from build123d import *

# Parameters (mm, degrees)
SKETCH1_W            = 75
SKETCH1_H            = 40
BOSS_EXTRUDE1_DEPTH  = 2
SKETCH2_W            = 75
SKETCH2_H            = 40
SKETCH2_W_2          = 71
SKETCH2_H_2          = 17
BOSS_EXTRUDE2_DEPTH  = 17
CUT_EXTRUDE2_DEPTH   = 17
CUT_EXTRUDE3_REACH   = 82.169
CUT_EXTRUDE4_REACH   = 88.683
SKETCH5_R            = 1.6
MIRROR2_COPY_1_DEPTH = 17
SKETCH7_W            = 80.259890461
SKETCH7_H            = 23.370696072
CUT_EXTRUDE5_DEPTH   = 19


with BuildPart() as part:
    # Sketch1 → Boss-Extrude1 (new body)
    with BuildSketch(Plane(origin=(0, 0, 0), x_dir=(1, 0, 0), z_dir=(0, 1, 0))):
        with Locations((37.5, 20)):
            Rectangle(SKETCH1_W, SKETCH1_H)
    boss_extrude1 = extrude(amount=BOSS_EXTRUDE1_DEPTH)

    # Sketch2 → Boss-Extrude2 (add)
    with BuildSketch(Plane(origin=(0, 2, 0), x_dir=(1, 0, 0), z_dir=(0, 1, 0))):
        with Locations((37.5, 20)):
            Rectangle(SKETCH2_W, SKETCH2_H)
        with Locations((37.5, 29.5)):
            Rectangle(SKETCH2_W_2, SKETCH2_H_2, mode=Mode.SUBTRACT)
        with Locations((37.5, 10.5)):
            Rectangle(SKETCH2_W_2, SKETCH2_H_2, mode=Mode.SUBTRACT)
    boss_extrude2 = extrude(amount=BOSS_EXTRUDE2_DEPTH)

    # Sketch3 → Cut-Extrude2 (cut)
    with BuildSketch(Plane.XY):
        with BuildLine():
            Line((2, 17.5), (2, 19))
            Line((2, 19), (73, 19))
            Line((73, 19), (73, 17.5))
            ThreePointArc((73, 17.5), (70.5, 15), (68, 17.5))
            Line((68, 17.5), (49, 17.5))
            Line((49, 17.5), (46, 15))
            Line((46, 15), (29, 15))
            Line((29, 15), (26, 17.5))
            Line((26, 17.5), (7, 17.5))
            ThreePointArc((7, 17.5), (4.5, 15), (2, 17.5))
        make_face()
    cut_extrude2 = extrude(amount=-CUT_EXTRUDE2_DEPTH, mode=Mode.SUBTRACT)

    # Mirror1: Cut-Extrude2 across plane
    add(cut_extrude2.mirror(Plane.XY.offset(-20)), mode=Mode.SUBTRACT)

    # Sketch4 → Cut-Extrude3 (cut, up to next)
    with BuildSketch(Plane.XY.offset(-19), mode=Mode.PRIVATE) as cut_extrude3_sk1:
        Polygon((2, 18), (7.035918341, 18), (10.035918341, 15), (64.964081659, 15), (67.964081659, 18), (73, 18), (73, 19), (2, 19), align=None)
    cut_extrude3_tool1 = extrude(cut_extrude3_sk1.sketch, amount=-CUT_EXTRUDE3_REACH, mode=Mode.PRIVATE) & part.part
    cut_extrude3 = cut_extrude3_tool1.solids().sort_by_distance((37.5, 17.098486, -19))[0]
    add(cut_extrude3, mode=Mode.SUBTRACT)

    # Sketch5 → Cut-Extrude4 (cut, up to next)
    with BuildSketch(Plane(origin=(0, 2, 0), x_dir=(1, 0, 0), z_dir=(0, 1, 0)), mode=Mode.PRIVATE) as cut_extrude4_sk1:
        with Locations(Location((37.5, 29.5, 0), (0, 0, 270))):
            Circle(SKETCH5_R)
    cut_extrude4_tool1 = extrude(cut_extrude4_sk1.sketch, amount=-CUT_EXTRUDE4_REACH, mode=Mode.PRIVATE) & part.part
    # Sketch5 → Cut-Extrude4 (cut, up to next)
    with BuildSketch(Plane(origin=(0, 2, 0), x_dir=(1, 0, 0), z_dir=(0, 1, 0)), mode=Mode.PRIVATE) as cut_extrude4_sk2:
        with Locations(Location((37.5, 10.5, 0), (0, 0, 270))):
            Circle(SKETCH5_R)
    cut_extrude4_tool2 = extrude(cut_extrude4_sk2.sketch, amount=-CUT_EXTRUDE4_REACH, mode=Mode.PRIVATE) & part.part
    cut_extrude4_1 = cut_extrude4_tool1.solids().sort_by_distance((37.5, 2, -29.5))[0]
    add(cut_extrude4_1, mode=Mode.SUBTRACT)
    cut_extrude4_2 = cut_extrude4_tool2.solids().sort_by_distance((37.5, 2, -10.5))[0]
    add(cut_extrude4_2, mode=Mode.SUBTRACT)
    cut_extrude4 = cut_extrude4_1 + cut_extrude4_2  # Cut-Extrude4 as one shape, for the pattern or mirror that repeats it

    # Mirror2: Boss-Extrude1, Boss-Extrude2, Cut-Extrude2, Cut-Extrude3, Cut-Extrude4 across plane
    add(boss_extrude1.mirror(Plane.XY.offset(-1)))
    add(boss_extrude2.mirror(Plane.XY.offset(-1)))
    add(cut_extrude2.mirror(Plane.XY.offset(-1)), mode=Mode.SUBTRACT)
    add(cut_extrude3.mirror(Plane.XY.offset(-1)), mode=Mode.SUBTRACT)
    add(cut_extrude4.mirror(Plane.XY.offset(-1)), mode=Mode.SUBTRACT)

    # Mirror2 copy 1 sketch → Mirror2 copy 1 (cut)
    with BuildSketch(Plane.XY.offset(38)):
        with BuildLine():
            Line((2, 17.5), (2, 19))
            Line((2, 19), (73, 19))
            Line((73, 19), (73, 17.5))
            ThreePointArc((73, 17.5), (70.5, 15), (68, 17.5))
            Line((68, 17.5), (49, 17.5))
            Line((49, 17.5), (46, 15))
            Line((46, 15), (29, 15))
            Line((29, 15), (26, 17.5))
            Line((26, 17.5), (7, 17.5))
            ThreePointArc((7, 17.5), (4.5, 15), (2, 17.5))
        make_face()
    extrude(amount=-MIRROR2_COPY_1_DEPTH, mode=Mode.SUBTRACT)

    # Sketch7 → Cut-Extrude5 (cut)
    with BuildSketch(Plane.XY.offset(38)):
        with Locations((37.807509159, 10.038141028)):
            Rectangle(SKETCH7_W, SKETCH7_H)
    extrude(amount=-CUT_EXTRUDE5_DEPTH, mode=Mode.SUBTRACT)


solid = part.part
For this review, take the finished solid that the model builds, in its own axes (mm). A direction names the side the tool comes from. Round coordinates to 2 decimals unless told otherwise and drop trailing zeros. Order: outer loops, then holes, each group sorted by start corner. A loop starts at its lowest first (then second) coordinate and runs counter-clockwise, first axis right, second up. Notation, with made-up numbers: M 65.5,51 L 81.5,51 A16 cw 81.5,80 Z; hole C -4.75,50 d4. An arc over 180 degrees is marked long. Use a Markdown table: item, result. Add a question column.
Item 1: Insertion check: pin 1 (0.6 mm diameter, centred on x = 62.5, z = -39, fed in from +Y); pin 2 (0.6 mm diameter, centred on x = 69.5, z = 18, fed in from +Y); pin 3 (8.5 mm diameter, centred on x = 51, z = -12.5, fed in from +Y). Each pin has a flat end and moves straight along its axis. Give the tip position at first contact, or say it passes through.
Item 2: Add section C-C, the plane z = -29.5. Give the boundary of the cut face in (x, y), then the cut area to 3 significant figures.
Item 3: Tool access review of faces 5 (the cylindrical face through (4.6, 15, -39)), 6 (the flat face through (66.443, 16.479, -19.986)), 7 (the cylindrical face through (35.94, 1.01, -29.85)), 8 (the flat face through (37, 7, -40)), 9 (the flat face through (70, 18, 18)): name each direction out of +Z, -Z, +X, -X, +Y, -Y from which nothing blocks a thin tool from reaching the whole face with its end or side.
Item 4: Add section D-D, the plane x = 4.5. Give the boundary of the cut face in (y, z).
Item 5: Add section B-B, the plane x = 37.5. Give the boundary of the cut face in (y, z).
Item 6: To check wall thickness, follow line 1 along Z through (x, y) = (71.5, 5); line 2 along X through (y, z) = (7, -5); line 3 along X through (y, z) = (1.45, -10.5). State the ranges of each line that lie inside material, in increasing order.
Item 7: Mouldability with a two-part tool opening along X and no side actions: class faces 1 (the flat face through (74, 19, -11)), 2 (the flat face through (75, 9, -10)), 3 (the flat face through (37, 10, -2)), 4 (the flat face through (37, 8, -21)) as released by +X, released by -X, zero draft, split by the parting line, or undercut.
Item 8: Add section A-A, the plane y = 10.5. Give the boundary of the cut face in (x, z), then the cut area to 3 significant figures.
Geometry results:
| question | item | result |
|---|---|---|
| 1 | pin 1 | stops at y = 17.5 |
| 1 | pin 2 | stops at y = 18 |
| 1 | pin 3 | stops at y = 2 |
| 2 | outline | M 0,0 L 35.9,0 L 35.9,2 L 2,2 L 2,19 L 0,19 Z; M 39.1,0 L 75,0 L 75,19 L 73,19 L 73,2 L 39.1,2 Z |
| 2 | area | 212 mm² |
| 3 | face 5 | -Z, +Y |
| 3 | face 6 | +Y |
| 3 | face 7 | +Y, -Y |
| 3 | face 8 | -Z, +X, -X, +Y, -Y |
| 3 | face 9 | +Z, -Z, +Y |
| 4 | outline | M 0,-40 L 15,-40 L 15,-38 L 2,-38 L 2,-21 L 18,-21 L 18,-19 L 2,-19 L 2,-2 L 15,-2 L 15,0 L 2,0 L 2,17 L 18,17 L 18,19 L 0,19 Z |
| 5 | outline | M 0,-40 L 15,-40 L 15,-38 L 2,-38 L 2,-31.1 L 0,-31.1 Z; M 0,-27.9 L 2,-27.9 L 2,-21 L 15,-21 L 15,-19 L 2,-19 L 2,-12.1 L 0,-12.1 Z; M 0,-8.9 L 2,-8.9 L 2,-2 L 15,-2 L 15,0 L 2,0 L 2,6.9 L 0,6.9 Z; M 0,10.1 L 2,10.1 L 2,17 L 15,17 L 15,19 L 0,19 Z |
| 6 | line 1 | z = -40 to -38, -21 to -19, -2 to 0, 17 to 19 |
| 6 | line 2 | x = 0 to 2, 73 to 75 |
| 6 | line 3 | x = 0 to 35.9, 39.1 to 75 |
| 7 | face 1 | zero draft |
| 7 | face 2 | released by +X |
| 7 | face 3 | undercut |
| 7 | face 4 | undercut |
| 8 | outline | M 0,-40 L 75,-40 L 75,19 L 0,19 Z; hole M 2,-38 L 73,-38 L 73,-21 L 2,-21 Z; hole M 2,-19 L 73,-19 L 73,-2 L 2,-2 Z; hole M 2,0 L 73,0 L 73,17 L 2,17 Z |
| 8 | area | 804 mm² |
